For this review, take the finished solid that the model builds, in its own axes (mm). A direction names the side the tool comes from. Round coordinates to 2 decimals unless told otherwise and drop trailing zeros. Write each loop counter-clockwise with the first axis right and the second up, starting at its lowest first coordinate (ties: lowest second). Pieces come first, ordered by that corner, then holes. Notation, with made-up numbers: (51.25, 24) -> (68.25, 24) arc R28 ccw to (68.25, 50) -> close; hole circle Ø8 at (4.5, -13.5). An arc over 180 degrees is marked (long way). Answer as CSV lines item,"result". Start each with the question number.
Item 1: Mouldability with a two-part tool opening along Y and no side actions: class faces 1 (the cylindrical face through (-8.801, -64.006, 3.131)), 2 (the flat face through (4, 1, 0)), 3 (the flat face through (-3.175, 42, 3)) as +Y half, -Y half, draft (parallel to the pull), parting line (faces both ways), or undercut.
Item 2: For pin 1 Ø5.5 at (x, y) = (0, -58.42) entering from -Z, flat-tipped, find the tip position at first contact; note if it passes through.
Item 3: Wall thickness on probe 1 along Y at (x, z) = (0, 4.5) (3 decimals); probe 2 along Y at (x, z) = (-1, 2.75); probe 3 along X at (y, z) = (45, 4.5) (3 decimals): over which ranges is each line inside the solid? List them lowest first. Write a range as from..to.
Item 4: Machinability: for faces 4 (the flat face through (0, 64.77, 3)), 5 (the flat face through (-3.81, -7, 3)), which of the approach directions +Z, -Z, +X, -X, +Y, -Y give a long, thin tool a straight path to every point of the face, cutting with its end or side? Answer none if there is none.
Item 5: Take a section at A-A on y = -58.42. Give the boundary of the cut face in (x, z) (3 decimals), then the cut area to 3 significant figures.
Item 6: Take a section at B-B on z = 4. Give the boundary of the cut face in (x, y) (3 decimals), then the cut area to 3 significant figures.
Item 7: Take a section at D-D on y = -28. Give the boundary of the cut face in (x, z) (3 decimals), then the cut area to 3 significant figures.
Item 8: Take a section at C-C on x = 0. Give the boundary of the cut face in (y, z) (3 decimals).
```python
from build123d import *

# Parameters (mm, degrees)
SKETCH1_R               = 3.175
BOSS_EXTRUDE1_DEPTH     = 6.35
CUT_EXTRUDE1_DEPTH      = 1
CUT_EXTRUDE1_DEPTH_BACK = 7.35
CUT_EXTRUDE2_DEPTH      = 7.35


with BuildPart() as part:
    # Sketch1 → Boss-Extrude1 (new body)
    with BuildSketch(Plane.XY):
        with BuildLine():
            Line((-6.985, -64.77), (6.985, -64.77))
            ThreePointArc((6.985, -64.77), (8.781051224, -64.026051224), (9.525, -62.23))
            Line((9.525, -62.23), (9.525, 64.77))
            Line((9.525, 64.77), (-9.525, 64.77))
            Line((-9.525, 64.77), (-9.525, -62.23))
            ThreePointArc((-9.525, -62.23), (-8.781051224, -64.026051224), (-6.985, -64.77))
        make_face()
        with Locations((0, -58.42)):
            Circle(SKETCH1_R, mode=Mode.SUBTRACT)
    extrude(amount=BOSS_EXTRUDE1_DEPTH)

    # Sketch2 → Cut-Extrude1 (cut, two sides)
    with BuildSketch(Plane.XY.offset(6.35)) as cut_extrude1_sk:
        with BuildLine():
            Line((-3.175, -41.91), (-3.175, 54.61))
            ThreePointArc((-3.175, 54.61), (0, 57.785), (3.175, 54.61))
            Line((3.175, 54.61), (3.175, -41.91))
            ThreePointArc((3.175, -41.91), (0, -45.085), (-3.175, -41.91))
        make_face()
    extrude(amount=CUT_EXTRUDE1_DEPTH, mode=Mode.SUBTRACT)
    extrude(cut_extrude1_sk.sketch, amount=-CUT_EXTRUDE1_DEPTH_BACK, mode=Mode.SUBTRACT)

    # Sketch3 → Cut-Extrude2 (cut, through all)
    with BuildSketch(Plane.XY.offset(6.35)):
        with BuildLine():
            Line((3.81, 28.098134356), (3.81, -41.91))
            ThreePointArc((3.81, -41.91), (0, -45.72), (-3.81, -41.91))
            Line((-3.81, -41.91), (-3.81, 28.098134356))
            ThreePointArc((-3.81, 28.098134356), (0, 31.908134356), (3.81, 28.098134356))
        make_face()
    extrude(amount=-CUT_EXTRUDE2_DEPTH, mode=Mode.SUBTRACT)


solid = part.part
```
Output values:
1,face 1,"-Y half"
1,face 2,"draft"
1,face 3,"undercut"
2,pin 1,"passes through"
3,probe 1,"y = -64.77..-61.595, -55.245..-45.72, 57.785..64.77"
3,probe 2,"y = -64.77..-61.43, -55.41..-45.59, 57.62..64.77"
3,probe 3,"x = -9.525..-3.175, 3.175..9.525"
4,face 4,"+Z, -Z, +X, -X, +Y"
4,face 5,"+Z, -Z"
5,outline,"(-9.525, 0) -> (-3.175, 0) -> (-3.175, 6.35) -> (-9.525, 6.35) -> close; (3.175, 0) -> (9.525, 0) -> (9.525, 6.35) -> (3.175, 6.35) -> close"
5,area,"80.6 mm^2"
6,outline,"(-9.525, -62.23) arc R2.54 ccw to (-6.985, -64.77) -> (6.985, -64.77) arc R2.54 ccw to (9.525, -62.23) -> (9.525, 64.77) -> (-9.525, 64.77) -> close; hole (-3.81, -41.91) arc R3.81 ccw to (3.81, -41.91) -> (3.81, 28.098) arc R3.81 ccw to (3.175, 30.204) -> (3.175, 54.61) arc R3.175 ccw to (-3.175, 54.61) -> (-3.175, 30.204) arc R3.81 ccw to (-3.81, 28.098) -> close; hole circle Ø6.35 at (0, -58.42)"
6,area,"1,690 mm^2"
7,outline,"(-9.525, 0) -> (-3.81, 0) -> (-3.81, 6.35) -> (-9.525, 6.35) -> close; (3.81, 0) -> (9.525, 0) -> (9.525, 6.35) -> (3.81, 6.35) -> close"
7,area,"72.6 mm^2"
8,outline,"(-64.77, 0) -> (-61.595, 0) -> (-61.595, 6.35) -> (-64.77, 6.35) -> close; (-55.245, 0) -> (-45.72, 0) -> (-45.72, 6.35) -> (-55.245, 6.35) -> close; (57.785, 0) -> (64.77, 0) -> (64.77, 6.35) -> (57.785, 6.35) -> close"
